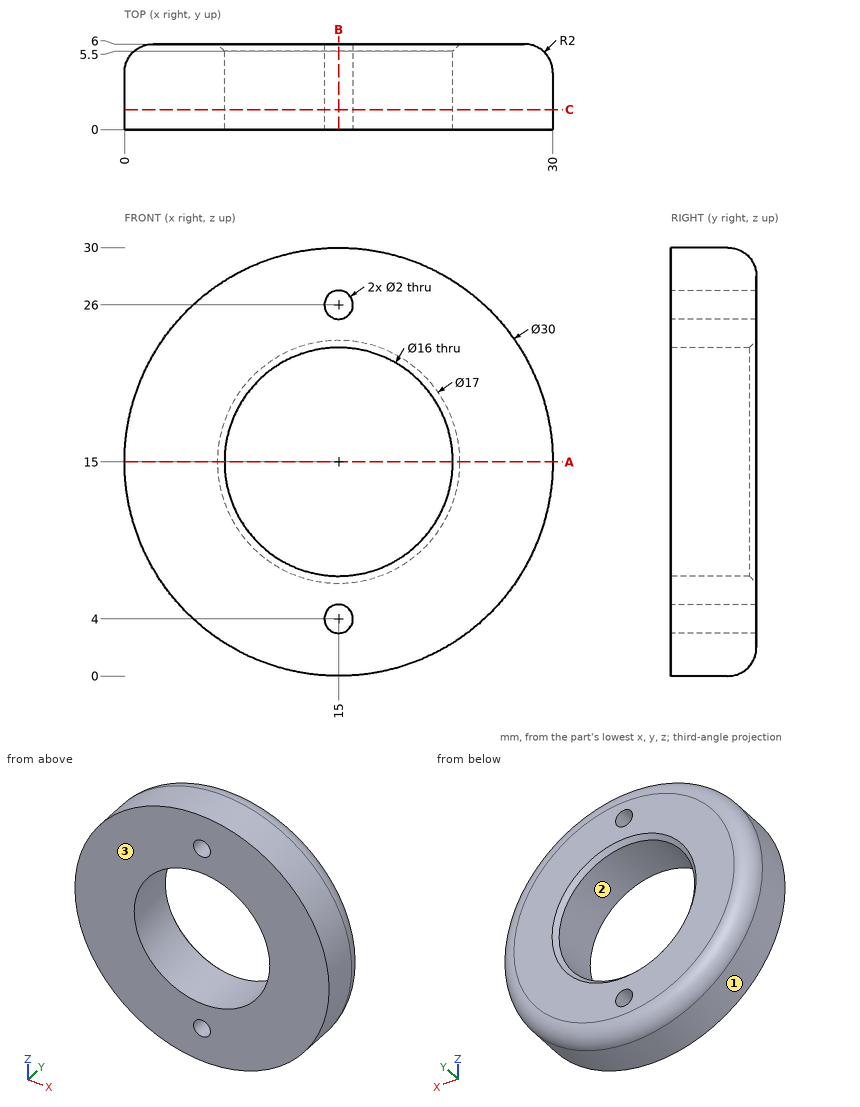
Answer from the drawing. Dimensions are ordinates in mm from the lowest x, y and z of the part. Give positions to 0.01 mm unless a question says otherwise; leave off trailing zeros. Loops run counter-clockwise (first coordinate to the right, second up) from the corner with the lowest first, then second, coordinate; pieces in that order, holes last. Notation, with made-up numbers: M -32,-29.5 L 9,-29.5 A34 ccw 9,5.5 Z; hole C -21,10 d6. An arc over 180 degrees is marked long. One line per item, written item: value.
Q1. Find the intervals of material crossed by line 1 (Z direction, x = 15, y = 4.1); line 2 (X direction, y = 2.7, z = 26); line 3 (X direction, y = 4.6, z = 26), in increasing order. Write a range as from..to.
Working result:
line 1: z = 0..3, 5..7, 23..25, 27..30
line 2: x = 4.8..14, 16..25.2
line 3: x = 4.94..14, 16..25.06
Q2. Flat-ended cylindrical pins translate along their axes: P1, Ø1.5, axis at x = 11, y = 0.5, coming from the +Z side; P2, Ø1.5, axis at y = 4, z = 25.5, coming from the +X side; P3, Ø1.5, axis at x = 4.5, y = 3.5, coming from the -Z side. Find the tip coordinate at first contact, or state that the pin passes through.
Working result:
P1: stops at z = 29.64
P2: stops at x = 26.4
P3: stops at z = 3.6
Q3. A cutting plane is placed at B-B on x = 15. Determine the outline of the cut face in (y, z).
Working result:
outline: M 0,0 L 4,0 A2 ccw 6,2 L 6,3 L 0,3 Z; M 0,5 L 6,5 L 6,6.5 L 5.5,7 L 0,7 Z; M 0,23 L 5.5,23 L 6,23.5 L 6,25 L 0,25 Z; M 0,27 L 6,27 L 6,28 A2 ccw 4,30 L 0,30 Z
Q4. A cutting plane is placed at C-C on y = 1.4. Determine the outline of the cut face in (x, z).
Working result:
outline: C 15,15 d30; hole C 15,15 d16; hole C 15,4 d2; hole C 15,26 d2
Q5. Determine the mould class of the marked faces 1, 2 and 3 for opening direction Z: +Z half, -Z half, draft (parallel to the pull), parting line (faces both ways), or undercut.
Working result:
face 1: parting line
face 2: undercut
face 3: draft
Q6. A cutting plane is placed at A-A on z = 15. Determine the outline of the cut face in (x, y), then the cut area to 3 significant figures.
Working result:
outline: M 0,0 L 7,0 L 7,5.5 L 6.5,6 L 2,6 A2 ccw 0,4 Z; M 23,0 L 30,0 L 30,4 A2 ccw 28,6 L 23.5,6 L 23,5.5 Z
area: 82.0 mm^2
